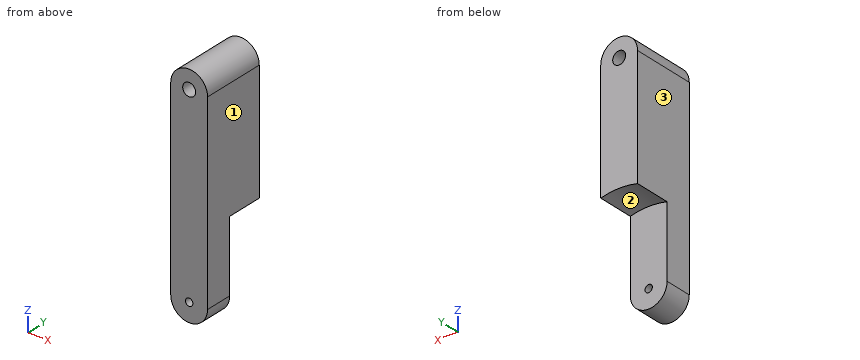
Autodesk Inventor part; units mm, degrees
ref_plane "YZ Plane" through (0, 0, 0) normal (1, 0, 0) x (0, 1, 0)
ref_plane "XZ Plane" through (0, 0, 0) normal (0, 1, 0) x (-1, 0, 0)
ref_plane "XY Plane" through (0, 0, 0) normal (0, 0, 1) x (1, 0, 0)
sketch "Sketch1" plane through (0, 0, 0) normal (0, 1, 0) x (-1, 0, 0)
  circle A0 centre (0, 0) radius 100
  line L0 (0, 0) -> (18.5658, -69.2885)
  line L1 (0, 0) -> (0, -103.5276)
  arc A1 (24.6448, -72.6673) -> (14.9907, -75.2542) centre (0, 0) ccw
  circle A2 centre (25.8819, -96.5926) radius 5
  arc A3 (24.729, -72.9816) -> (15.0747, -75.5678) centre (19.8599, -74.1181) ccw
  line L2 (30.6777, -95.1782) -> (24.6448, -72.6673)
  line L3 (21.0523, -97.8867) -> (14.9907, -75.2542)
  circle A4 centre (0, -103.5276) radius 11.6229
  line L4 (21.0523, -97.8867) -> (25.8819, -96.5926)
  arc A5 (-25.8819, -96.5926) -> (26.7197, -101.5219) centre (0, -103.5276) ccw
  circle A6 centre (0, -103.5276) radius 40
  arc A7 (57.9067, -50.8394) -> (50.8389, -57.9063) centre (54.2582, -54.2582) ccw
  line L5 (67.1751, -74.2462) -> (50.6094, -57.6767)
  line L6 (74.1567, -67.0879) -> (57.6767, -50.6094)
  circle A8 centre (70.7107, -70.7107) radius 5
  circle A9 centre (51.7638, -89.6575) radius 11.6229
  arc A10 (75.5684, -15.0748) -> (72.9809, -24.7289) centre (74.1181, -19.8599) ccw
  line L7 (95.2985, -30.7115) -> (72.6673, -24.6448)
  line L8 (97.7655, -21.0214) -> (75.2542, -14.9907)
  circle A11 centre (96.5926, -25.8819) radius 5
  circle A12 centre (89.6575, -51.7638) radius 11.6229
  arc A13 (72.9816, 24.729) -> (75.5678, 15.0747) centre (74.1181, 19.8599) ccw
  line L9 (97.8867, 21.0523) -> (75.2542, 14.9907)
  line L10 (95.1782, 30.6777) -> (72.6673, 24.6448)
  circle A14 centre (96.5926, 25.8819) radius 5
  circle A15 centre (103.5276, 0) radius 11.6229
  arc A16 (50.8394, 57.9067) -> (57.9063, 50.8389) centre (54.2582, 54.2582) ccw
  line L11 (74.2462, 67.1751) -> (57.6767, 50.6094)
  line L12 (67.0879, 74.1567) -> (50.6094, 57.6767)
  circle A17 centre (70.7107, 70.7107) radius 5
  circle A18 centre (89.6575, 51.7638) radius 11.6229
  arc A19 (15.0748, 75.5684) -> (24.7289, 72.9809) centre (19.8599, 74.1181) ccw
  line L13 (30.7115, 95.2985) -> (24.6448, 72.6673)
  line L14 (21.0214, 97.7655) -> (14.9907, 75.2542)
  circle A20 centre (25.8819, 96.5926) radius 5
  circle A21 centre (51.7638, 89.6575) radius 11.6229
  arc A22 (-24.729, 72.9816) -> (-15.0747, 75.5678) centre (-19.8599, 74.1181) ccw
  line L15 (-21.0523, 97.8867) -> (-14.9907, 75.2542)
  line L16 (-30.6777, 95.1782) -> (-24.6448, 72.6673)
  circle A23 centre (-25.8819, 96.5926) radius 5
  circle A24 centre (0, 103.5276) radius 11.6229
  arc A25 (-57.9067, 50.8394) -> (-50.8389, 57.9063) centre (-54.2582, 54.2582) ccw
  line L17 (-67.1751, 74.2462) -> (-50.6094, 57.6767)
  line L18 (-74.1567, 67.0879) -> (-57.6767, 50.6094)
  circle A26 centre (-70.7107, 70.7107) radius 5
  circle A27 centre (-51.7638, 89.6575) radius 11.6229
  arc A28 (-75.5684, 15.0748) -> (-72.9809, 24.7289) centre (-74.1181, 19.8599) ccw
  line L19 (-95.2985, 30.7115) -> (-72.6673, 24.6448)
  line L20 (-97.7655, 21.0214) -> (-75.2542, 14.9907)
  circle A29 centre (-96.5926, 25.8819) radius 5
  circle A30 centre (-89.6575, 51.7638) radius 11.6229
  arc A31 (-72.9816, -24.729) -> (-75.5678, -15.0747) centre (-74.1181, -19.8599) ccw
  line L21 (-97.8867, -21.0523) -> (-75.2542, -14.9907)
  line L22 (-95.1782, -30.6777) -> (-72.6673, -24.6448)
  circle A32 centre (-96.5926, -25.8819) radius 5
  circle A33 centre (-103.5276, 0) radius 11.6229
  arc A34 (-50.8394, -57.9067) -> (-57.9063, -50.8389) centre (-54.2582, -54.2582) ccw
  line L23 (-74.2462, -67.1751) -> (-57.6767, -50.6094)
  line L24 (-67.0879, -74.1567) -> (-50.6094, -57.6767)
  circle A35 centre (-70.7107, -70.7107) radius 5
  circle A36 centre (-89.6575, -51.7638) radius 11.6229
  arc A37 (-15.0748, -75.5684) -> (-24.7289, -72.9809) centre (-19.8599, -74.1181) ccw
  line L25 (-30.7115, -95.2985) -> (-24.6448, -72.6673)
  line L26 (-21.0214, -97.7655) -> (-14.9907, -75.2542)
  circle A38 centre (-25.8819, -96.5926) radius 5
  circle A39 centre (-51.7638, -89.6575) radius 11.6229
  circle A40 centre (0, 0) radius 3.5
  circle A41 centre (0, -103.5276) radius 2
  circle A42 centre (0, 0) radius 10
  circle A43 centre (0, -103.5276) radius 10
  line L27 (10, 0) -> (10, -103.5276)
  line L28 (-10, 0) -> (-10, -103.5276)
  point P0 (50.7227, -50.7227)
  point P1 (73.9009, -74.5607)
  point P2 (69.2885, -18.5658)
  point P3 (101.2804, -27.621)
  point P4 (69.2885, 18.5658)
  point P5 (101.5219, 26.7197)
  point P6 (50.7227, 50.7227)
  point P7 (74.5607, 73.9009)
  point P8 (18.5658, 69.2885)
  point P9 (27.621, 101.2804)
  point P10 (-18.5658, 69.2885)
  point P11 (-26.7197, 101.5219)
  point P12 (-50.7227, 50.7227)
  point P13 (-73.9009, 74.5607)
  point P14 (-69.2885, 18.5658)
  point P15 (-101.2804, 27.621)
  point P16 (-69.2885, -18.5658)
  point P17 (-101.5219, -26.7197)
  point P18 (-50.7227, -50.7227)
  point P19 (-74.5607, -73.9009)
  point P20 (-18.5658, -69.2885)
  point P21 (-27.621, -101.2804)
  point P22 (40.2917, -91.5236)
  point P23 (59.1159, -80.6555)
  point P24 (67.0867, -74.1578)
  point P25 (80.6555, -59.1159)
  point P26 (91.5236, -40.2917)
  point P27 (95.1777, -30.6791)
  point P28 (99.4077, -10.8682)
  point P29 (99.4077, 10.8682)
  point P30 (97.7659, 21.0199)
  point P31 (91.5236, 40.2917)
  point P32 (80.6555, 59.1159)
  point P33 (74.1578, 67.0867)
  point P34 (59.1159, 80.6555)
  point P35 (40.2917, 91.5236)
  point P36 (30.6791, 95.1777)
  point P37 (10.8682, 99.4077)
  point P38 (-10.8682, 99.4077)
  point P39 (-21.0199, 97.7659)
  point P40 (-40.2917, 91.5236)
  point P41 (-59.1159, 80.6555)
  point P42 (-67.0867, 74.1578)
  point P43 (-80.6555, 59.1159)
  point P44 (-91.5236, 40.2917)
  point P45 (-95.1777, 30.6791)
  point P46 (-99.4077, 10.8682)
  point P47 (-99.4077, -10.8682)
  point P48 (-97.7659, -21.0199)
  point P49 (-91.5236, -40.2917)
  point P50 (-80.6555, -59.1159)
  point P51 (-74.1578, -67.0867)
  point P52 (-59.1159, -80.6555)
  point P53 (-40.2917, -91.5236)
  point P54 (-30.6791, -95.1777)
  point P55 (-10.8682, -99.4077)
  point P56 (10.8682, -99.4077)
  point P57 (21.0199, -97.7659)
  point P58 (-10, -64.7978)
  point P59 (10, -64.7978)
  dimension "d2" = 200
  dimension "d3" = 15
  dimension "d4" = 10
  dimension "d5" = 10
  dimension "d6" = 80
  dimension "d7" = 360
  dimension "d8" = 7
  dimension "d9" = 4
  dimension "d10" = 20
  dimension "d11" = 20
extrude "Extrusion1" add sketch "Sketch1" along normal blind 20 contours L28 A42 L1 A6 | L1 A42 L0 L27 A6 | A42 L0 A40 L1 | L1 A40 L0 A42 | L27 L0 A42
extrude "Extrusion2" add sketch "Sketch1" against normal blind 15 contours L28 A4 L1 A43 A0 | A0 A43 L28 | L28 A1 L1 A4 | A43 L1 A0 | A0 A43 | A4 L27 A0 A43 L1 | L1 A1 L27 A4 | L28 A6 L1 A1 | L1 A43 A0 | A43 A0 L27 | L1 A6 L27 A1 | L28 A42 L1 A6 | L1 A42 L0 L27 A6 | A42 L0 A40 L1 | L1 A40 L0 A42 | L27 L0 A42
properties part number "SC-1-02-Bridge"
Part model, mm, in its own coordinate system. Face numbers are marked on the shaded views. Round coordinates to 2 decimals unless told otherwise and drop trailing zeros. Loops run counter-clockwise (first coordinate to the right, second up) from the corner with the lowest first, then second, coordinate; pieces in that order, holes last.
Item 1: Drop a flat-ended pin along its axis: P1, Ø5, axis at x = -4.5, y = -5.5, coming from the +Z side. Give the stop position or say it passes through.
Item 2: Cut at C-C, the plane y = 4. Give the cut face in (x, z), then the cut area to 3 significant figures.
Item 3: Cut at B-B, the plane y = -7.5. Give the cut face in (x, z), then the cut area to 3 significant figures.
Item 4: Drill centre lines: line 1 (Z direction, x = 0, y = -5.75); line 2 (Z direction, x = 0, y = 9); line 3 (Z direction, x = -1, y = -10). Where is each one in solid material? Low to high.
Item 5: Mould opens along X. For the marked faces 1, 2 and 3 say: +X half, -X half, draft (parallel to the pull), parting line (faces both ways), or undercut.
Item 6: Cut at A-A, the plane x = 0. Give the cut face in (y, z).
Item 7: Cut at D-D, the plane z = -86. Give the cut face in (x, y), then the cut area to 3 significant figures.
A:
1. P1: stops at z = 9.8
2. outline: (-10, -64.8) arc R40 cw to (10, -64.8) - (10, 0) arc R10 ccw to (-10, 0) - close; hole circle Ø7 at (0, 0)
2. area: 1,400 mm2
3. outline: (-10, -103.53) arc R10 ccw to (10, -103.53) - (10, 0) arc R10 ccw to (-10, 0) - close; hole circle Ø7 at (0, 0); hole circle Ø4 at (0, -103.53)
3. area: 2,330 mm2
4. line 1: z = -113.53 to -105.53, -101.53 to -3.5, 3.5 to 10
4. line 2: z = -63.53 to -3.5, 3.5 to 10
4. line 3: z = -113.48 to -105.26, -101.8 to -3.35, 3.35 to 9.95
5. face 1: +X half
5. face 2: undercut
5. face 3: -X half
6. outline: (-15, -113.53) - (0, -113.53) - (0, -105.53) - (-15, -105.53) - close; (-15, -101.53) - (0, -101.53) - (0, -63.53) - (20, -63.53) - (20, -3.5) - (-15, -3.5) - close; (-15, 3.5) - (20, 3.5) - (20, 10) - (-15, 10) - close
7. outline: (-10, -15) - (10, -15) - (10, 0) - (-10, 0) - close
7. area: 300 mm2
